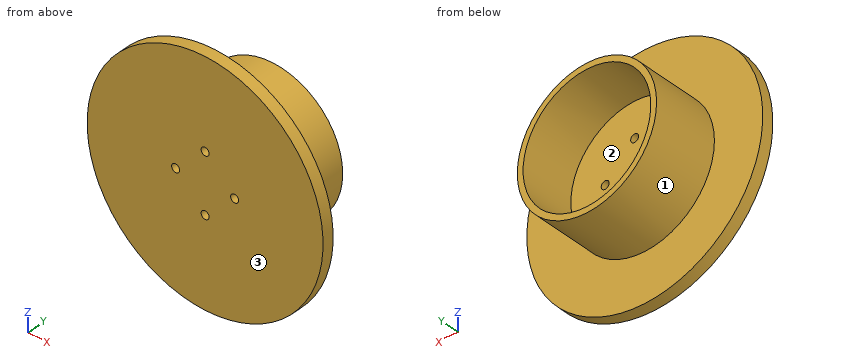
from build123d import *

# Parameters (mm, degrees)
SKETCH1_R           = 19.1875
BOSS_EXTRUDE1_DEPTH = 3.175
SKETCH2_R           = 19.1875
SKETCH2_R_2         = 17.6
BOSS_EXTRUDE2_DEPTH = 15
SKETCH3_R           = 1.1
CUT_EXTRUDE1_DEPTH  = 33.659622434
BOSS_EXTRUDE3_START = 3.175
SKETCH4_R           = 32.5
SKETCH4_R_2         = 1.1
BOSS_EXTRUDE3_DEPTH = 3.175


with BuildPart() as part:
    # Sketch1 → Boss-Extrude1 (new body)
    with BuildSketch(Plane(origin=(0, 0, 0), x_dir=(1, 0, 0), z_dir=(0, 1, 0))):
        with Locations(Location((0, 0, 0), (0, 0, 270))):
            Circle(SKETCH1_R)
    extrude(amount=BOSS_EXTRUDE1_DEPTH)

    # Sketch2 → Boss-Extrude2 (add)
    with BuildSketch(Plane(origin=(0, 3.175, 0), x_dir=(1, 0, 0), z_dir=(0, 1, 0))):
        with Locations(Location((0, 0, 0), (0, 0, 270))):
            Circle(SKETCH2_R)
        with Locations(Location((0, 0, 0), (0, 0, 270))):
            Circle(SKETCH2_R_2, mode=Mode.SUBTRACT)
    extrude(amount=BOSS_EXTRUDE2_DEPTH)

    # Sketch3 → Cut-Extrude1 (cut, through all)
    with BuildSketch(Plane.XZ):
        with Locations(Location((0, 8.125, 0), (0, 0, 270))):
            Circle(SKETCH3_R)
        with Locations(Location((8.125, 0, 0), (0, 0, 270))):
            Circle(SKETCH3_R)
        with Locations(Location((-8.125, 0, 0), (0, 0, 270))):
            Circle(SKETCH3_R)
        with Locations(Location((0, -8.125, 0), (0, 0, 270))):
            Circle(SKETCH3_R)
    extrude(amount=-CUT_EXTRUDE1_DEPTH, mode=Mode.SUBTRACT)

    # Sketch4 → Boss-Extrude3 (add)
    with BuildSketch(Plane.XZ.offset(BOSS_EXTRUDE3_START)):
        with Locations(Location((0, 0, 0), (0, 0, 270))):
            Circle(SKETCH4_R)
        with Locations(Location((0, -8.125, 0), (0, 0, 270))):
            Circle(SKETCH4_R_2, mode=Mode.SUBTRACT)
        with Locations(Location((8.125, 0, 0), (0, 0, 270))):
            Circle(SKETCH4_R_2, mode=Mode.SUBTRACT)
        with Locations(Location((-8.125, 0, 0), (0, 0, 270))):
            Circle(SKETCH4_R_2, mode=Mode.SUBTRACT)
        with Locations(Location((0, 8.125, 0), (0, 0, 270))):
            Circle(SKETCH4_R_2, mode=Mode.SUBTRACT)
    extrude(amount=-BOSS_EXTRUDE3_DEPTH)


solid = part.part
Can you work these out from the model? Positions are in its coordinate system, mm. Face numbers are marked on the shaded views. Coordinates: 2 decimals unless noted, no trailing zeros. Loops run counter-clockwise (first coordinate to the right, second up) from the corner with the lowest first, then second, coordinate; pieces in that order, holes last. Notation, with made-up numbers: (-1, 56) - (36, 56) arc R13 ccw to (36, 61) - close; hole circle Ø3 at (67.25, 65.25). An arc over 180 degrees is marked (long way). Put each result on its own line as item: value. Start each with the question number.
Item 1: If I drill on line 1 along X through (y, z) = (-0.75, 0) (3 decimals); line 2 along X through (y, z) = (0.5, 0) (1 decimal); line 3 along Y through (x, z) = (-12, -28.5) (3 decimals), over which ranges is the centre line in solid material (lowest first)?
Item 2: Suppose I cut it at C-C (y = 13.5). Please give me the cut outline in (x, z) (1 decimal).
Item 3: Suppose I cut it at D-D (z = -13). Please give me the cut outline in (x, y) (3 decimals).
Item 4: Suppose I cut it at A-A (z = 0). Please give me the cut outline in (x, y) (1 decimal).
Item 5: If we mould it in two halves opening along X, with no side actions, what happens to the marked faces 1, 2 and 3? For each: +X half, -X half, draft (parallel to the pull), parting line (faces both ways), or undercut.
Item 6: Suppose I cut it at B-B (x = 0). Please give me the cut outline in (y, z) (1 decimal), and give its area (3 significant figures).
Item 7: For pin 1 (3 mm diameter, centred on x = 8.5, y = 7.5, fed in from -Z); pin 2 (5 mm diameter, centred on x = -11.5, y = 9, fed in from -Z); pin 3 (4 mm diameter, centred on x = -13.5, y = 12.5, fed in from -Z), each with a flat end and sliding along its axis, tell me the tip position at first contact or that it passes through.
Here are the results:
1. line 1: -32.5 to -9.225, -7.025 to 7.025, 9.225 to 32.5
1. line 2: -19.2 to -9.2, -7 to 7, 9.2 to 19.2
1. line 3: -3.175 to 0
2. outline: circle Ø38.4 at (0, 0); hole circle Ø35.2 at (0, 0)
3. outline: (-29.787, -3.175) - (29.787, -3.175) - (29.787, 0) - (14.112, 0) - (14.112, 18.175) - (11.864, 18.175) - (11.864, 3.175) - (-11.864, 3.175) - (-11.864, 18.175) - (-14.112, 18.175) - (-14.112, 0) - (-29.787, 0) - close
4. outline: (-32.5, -3.2) - (-9.2, -3.2) - (-9.2, 3.2) - (-17.6, 3.2) - (-17.6, 18.2) - (-19.2, 18.2) - (-19.2, 0) - (-32.5, 0) - close; (-7, -3.2) - (7, -3.2) - (7, 3.2) - (-7, 3.2) - close; (9.2, -3.2) - (32.5, -3.2) - (32.5, 0) - (19.2, 0) - (19.2, 18.2) - (17.6, 18.2) - (17.6, 3.2) - (9.2, 3.2) - close
5. face 1: parting line
5. face 2: undercut
5. face 3: draft
6. outline: (-3.2, -32.5) - (0, -32.5) - (0, -19.2) - (18.2, -19.2) - (18.2, -17.6) - (3.2, -17.6) - (3.2, -9.2) - (-3.2, -9.2) - close; (-3.2, -7) - (3.2, -7) - (3.2, 7) - (-3.2, 7) - close; (-3.2, 9.2) - (3.2, 9.2) - (3.2, 17.6) - (18.2, 17.6) - (18.2, 19.2) - (0, 19.2) - (0, 32.5) - (-3.2, 32.5) - close
6. area: 348 mm²
7. pin 1: z = -17.87
7. pin 2: z = -16.95
7. pin 3: z = -15.36
